Verification items for the finished model (mm, model axes). A direction names the side the tool comes from. Give positions to 0.01 mm unless a question says otherwise; leave off trailing zeros. Loops run counter-clockwise (first coordinate to the right, second up) from the corner with the lowest first, then second, coordinate; pieces in that order, holes last. Notation, with made-up numbers: M 42.25,-4.75 L 46.25,-4.75 A27 ccw 46.25,22.25 Z; hole C 36,67.25 d10. An arc over 180 degrees is marked long. Answer in a Markdown table with one row per item.
```python
from build123d import *

# Parameters (mm, degrees)
SKETCH1_R           = 2.5
SKETCH1_R_2         = 3
BOSS_EXTRUDE1_DEPTH = 6.2


with BuildPart() as part:
    # Sketch1 → Boss-Extrude1 (new body)
    with BuildSketch(Plane.XY):
        with BuildLine():
            Line((85.6, -33.2), (-2.718519223, -20.878508118))
            ThreePointArc((-2.718519223, -20.878508118), (-8.41017463, -20.715920511), (-14, -21.8))
            Line((-14, -21.8), (-42.039824529, -38.092696265))
            ThreePointArc((-42.039824529, -38.092696265), (-46.884666341, -40.111316958), (-52.087842039, -40.8))
            Line((-52.087842039, -40.8), (-81.699109919, -40.8))
            ThreePointArc((-81.699109919, -40.8), (-91.370795398, -43.36753119), (-98.495572761, -50.394))
            ThreePointArc((-98.495572761, -50.394), (-129.24406218, -50.82175889), (-115.5, -23.312608885))
            Line((-115.5, -23.312608885), (-95.618089435, -21.65))
            ThreePointArc((-95.618089435, -21.65), (-78.309182519, -16.601252711), (-64.341378668, -5.2))
            ThreePointArc((-64.341378668, -5.2), (-61.413749232, -2.21456762), (-58, 0.2))
            ThreePointArc((-58, 0.2), (-29.282001226, 11.518177334), (1.5, 13.818827736))
            ThreePointArc((1.5, 13.818827736), (139.454874424, 0.958251967), (274.87829908, -28.323787594))
            ThreePointArc((274.87829908, -28.323787594), (283.738974288, -51.630641354), (258.857280718, -53.25))
            ThreePointArc((258.857280718, -53.25), (172.558903288, -40.371111866), (85.6, -33.2))
        make_face()
        with Locations(Location((-114, -41.25, 0), (0, 0, 180))):
            Circle(SKETCH1_R, mode=Mode.SUBTRACT)
        with Locations(Location((270.7, -43.25, 0), (0, 0, 180))):
            Circle(SKETCH1_R, mode=Mode.SUBTRACT)
        with Locations(Location((-47, -18.8, 0), (0, 0, 180))):
            Circle(SKETCH1_R_2, mode=Mode.SUBTRACT)
        with Locations(Location((45.6, -19.2, 0), (0, 0, 180))):
            Circle(SKETCH1_R_2, mode=Mode.SUBTRACT)
        with Locations(Location((0, 0, 0), (0, 0, 180))):
            Circle(SKETCH1_R_2, mode=Mode.SUBTRACT)
        with BuildLine():
            ThreePointArc((226.744224082, -27.259797753), (211.929816899, -23.860779344), (197.071572094, -20.658819377))
            ThreePointArc((197.071572094, -20.658819377), (190.434794526, -25.546132018), (195.40651845, -32.119913468))
            ThreePointArc((195.40651845, -32.119913468), (210.197393834, -34.160215491), (224.964543777, -36.365688118))
            ThreePointArc((224.964543777, -36.365688118), (230.232403999, -32.668395241), (226.744224082, -27.259797753))
        make_face(mode=Mode.SUBTRACT)
        with BuildLine():
            ThreePointArc((132.347185699, -9.089339403), (122.571709195, -15.840894216), (130.010518711, -25.104130489))
            ThreePointArc((130.010518711, -25.104130489), (147.296090717, -26.642266435), (164.560225388, -28.404797523))
            ThreePointArc((164.560225388, -28.404797523), (172.152990765, -22.51669502), (166.534944909, -14.721991823))
            ThreePointArc((166.534944909, -14.721991823), (149.462384392, -11.776267989), (132.347185699, -9.089339403))
        make_face(mode=Mode.SUBTRACT)
    extrude(amount=BOSS_EXTRUDE1_DEPTH)


solid = part.part
```
Item 1: Sectioned sample at A-A (z = 1). Record the cut outline in (x, y).
Reported:
| item | result |
|---|---|
| outline | M -115.5,-23.31 A18 ccw long -98.5,-50.39 A19.5 cw -81.7,-40.8 L -52.09,-40.8 A20 ccw -42.04,-38.09 L -14,-21.8 A25.92 cw -2.72,-20.88 L 85.6,-33.2 A1325 cw 258.86,-53.25 A15.5 ccw long 274.88,-28.32 A1155.37 ccw 1.5,13.82 A103 ccw -58,0.2 A23.32 ccw -64.34,-5.2 A45.29 cw -95.62,-21.65 Z; hole C -114,-41.25 d5; hole C -47,-18.8 d6; hole C 0,0 d6; hole C 45.6,-19.2 d6; hole M 130.01,-25.1 A1336 cw 164.56,-28.4 A6.92 ccw 166.53,-14.72 A1144.37 ccw 132.35,-9.09 A8.11 ccw long Z; hole M 195.41,-32.12 A1336 cw 224.96,-36.37 A4.64 ccw 226.74,-27.26 A1144.37 ccw 197.07,-20.66 A5.79 ccw long Z; hole C 270.7,-43.25 d5 |
Item 2: Release check for a two-part mould opening along Y. For faces 1 (the flat face through (42.059, -27.126, 3.057)), 2 (the cylindrical face through (122.6, -15.66, 3.06)), 3 (the cylindrical face through (-78.5, -16.7, 3.1)) record: released by +Y, released by -Y, zero draft, split by the parting line, or undercut.
Reported:
| item | result |
|---|---|
| face 1 | released by -Y |
| face 2 | undercut |
| face 3 | released by +Y |
Item 3: Tool access check on faces 4 (the cylindrical face through (-91.25, -43.3, 3.06)), 5 (the cylindrical face through (137.54, 1.25, 3.06)), 6 (the cylindrical face through (172.13, -22.66, 3.06)). Record the directions out of +Z, -Z, +X, -X, +Y, -Y that give a thin tool (end or side, any length) a straight path to the whole face; none if there is none.
Reported:
| item | result |
|---|---|
| face 4 | +Z, -Z, -Y |
| face 5 | +Z, -Z, +X, +Y |
| face 6 | +Z, -Z |
Item 4: Sectioned sample at B-B (x = 150.5). Record the cut outline in (y, z), and give its area (3 significant figures).
Reported:
| item | result |
|---|---|
| outline | M -38.01,0 L -26.95,0 L -26.95,6.2 L -38.01,6.2 Z; M -11.95,0 L -0.8,0 L -0.8,6.2 L -11.95,6.2 Z |
| area | 138 mm^2 |
Item 5: Go/stop test with flat-tipped pins: pin 1 (1 mm diameter, centred on x = -41.5, z = 4, fed in from +Y); pin 2 (5 mm diameter, centred on x = 45.6, y = -19.2, fed in from -Z) (1 decimal). Record where each tip stops, or that it passes through.
Reported:
| item | result |
|---|---|
| pin 1 | stops at y = 8.09 |
| pin 2 | passes through |
Item 6: Scan lines: L1, parallel to Y at x = -14, z = 4; L2, parallel to Y at x = -47, z = 3.75; L3, parallel to Y at x = 196, z = 3.75. Record each from-to range of solid material in increasing order. Write a range as [from, to].
Reported:
| item | result |
|---|---|
| L1 | y = [-21.8, 13.83] |
| L2 | y = [-40.14, -21.8], [-15.8, 5.73] |
| L3 | y = [-43.3, -32.2], [-20.59, -9.2] |
